Source: CAD feature listing. Evaluate the final solid. Frame: model axes, mm. Face numbers are marked on the shaded views. A direction names the side the tool comes from. Give positions to 0.01 mm unless a question says otherwise; leave off trailing zeros. Loops run counter-clockwise (first coordinate to the right, second up) from the corner with the lowest first, then second, coordinate; pieces in that order, holes last. Notation, with made-up numbers: (46.25, 6) -> (74.25, 6) arc R18 ccw to (74.25, 32) -> close; hole circle Ø5 at (89.5, 66.5). An arc over 180 degrees is marked (long way). Return JSON: item names as keys, results as strings. Group by question number.
(1) Cut plane D-D on z = 14. Give the number of separate pieces and of enclosed holes in the cut face, then the cut area to 3 significant figures.
(2) Cut plane A-A on z = 0. Return loops of the section in (x, y) (3 decimals), then the cut area to 3 significant figures.
(3) Cut plane C-C on z = -3.5. Return loops of the section in (x, y) (3 decimals), then the cut area to 3 significant figures.
(4) Ray query, line 1 (Z direction, x = -13.5, y = 1); line 2 (Z direction, x = -4.5, y = 1); line 3 (Y direction, x = -9, z = 14) (3 decimals). Return the intervals inside material, ascending. Write a range as from..to.
(5) Cut plane B-B on x = 0. Return loops of the section in (y, z) (3 decimals).
(6) Pin query (flat end, axial travel): pin 1 (1.6 mm diameter, centred on x = 3.5, y = 1, fed in from -Z); pin 2 (1.6 mm diameter, centred on x = 13.47, z = 13.47, fed in from -Y); pin 3 (5 mm diameter, centred on x = -2, z = 5, fed in from +Y) (3 decimals). Return the tip coordinate at first contact, or that it passes through.
(7) Access query for the marked faces 1 and 2. Directions: +Z, -Z, +X, -X, +Y, -Y. A direction counts if a zero-diameter tool reaches every point of the face in a straight line with its end or side. Return the directions, or none.
(8) Draft query along X for the marked faces 3, 4 and 5. Return one class per face: released by +X, released by -X, zero draft, split by the parting line, or undercut.
```python
from build123d import *

# Parameters (mm, degrees)
SKETCH1_W                   = 33.528
SKETCH1_H                   = 33.02
BOSS_EXTRUDE1_DEPTH         = 3.175
CUT_EXTRUDE1_DEPTH          = 24.742207585
CUT_EXTRUDE2_DEPTH          = 24.742207585
SKETCH4_W                   = 6.08076
SKETCH4_H                   = 5.45338
BOSS_EXTRUDE2_DEPTH         = 6.08076
SKETCH5_W                   = 6.08076
SKETCH5_H                   = 5.45338
BOSS_EXTRUDE3_DEPTH         = 6.08076
SKETCH6_W                   = 6.08076
SKETCH6_H                   = 5.45338
BOSS_EXTRUDE4_DEPTH         = 6.08076
SKETCH7_W                   = 6.08076
SKETCH7_H                   = 5.45338
BOSS_EXTRUDE5_DEPTH         = 6.08076
HOLE1_D                     = 12.7254
M2_5_CLEARANCE_HOLE1_D      = 2.7051
M3_CLEARANCE_HOLE1_D        = 3.556
M2_5_CLEARANCE_HOLE2_D      = 2.7051
M2_5_CLEARANCE_HOLE2_DEPTH  = 39.60876
M2_5_CLEARANCE_HOLE3_D      = 2.7051
M2_5_CLEARANCE_HOLE3_DEPTH  = 39.60876
M2_5_CLEARANCE_HOLE4_REACH  = 27.061
M2_5_CLEARANCE_HOLE4_BORE_R = 1.35255
FILLET1_R                   = 0.635
FILLET2_R                   = 3.04038
CUT_EXTRUDE3_REACH          = 26.153


with BuildPart() as part:
    # Sketch1 → Boss-Extrude1 (new body)
    with BuildSketch(Plane(origin=(0, 3.175, 0), x_dir=(1, 0, 0), z_dir=(0, 1, 0))):
        Rectangle(SKETCH1_W, SKETCH1_H)
    extrude(amount=-BOSS_EXTRUDE1_DEPTH)

    # Sketch2 → Cut-Extrude1 (cut, through all)
    with BuildSketch(Plane.XZ):
        with BuildLine():
            Line((16.764, -10.42924), (16.764, 10.42924))
            ThreePointArc((16.764, 10.42924), (14.617411383, 9.536940757), (13.7287, 7.388864244))
            Line((13.7287, 7.388864244), (13.7287, -7.388864244))
            ThreePointArc((13.7287, -7.388864244), (14.617411383, -9.536940757), (16.764, -10.42924))
        make_face()
    extrude(amount=-CUT_EXTRUDE1_DEPTH, mode=Mode.SUBTRACT)

    # Sketch3 → Cut-Extrude2 (cut, through all)
    with BuildSketch(Plane.XZ):
        with BuildLine():
            Line((-16.764, 10.42924), (-16.764, -10.42924))
            ThreePointArc((-16.764, -10.42924), (-14.617411383, -9.536940757), (-13.7287, -7.388864244))
            Line((-13.7287, -7.388864244), (-13.7287, 7.388864244))
            ThreePointArc((-13.7287, 7.388864244), (-14.617411383, 9.536940757), (-16.764, 10.42924))
        make_face()
    extrude(amount=-CUT_EXTRUDE2_DEPTH, mode=Mode.SUBTRACT)

    # Sketch4 → Boss-Extrude2 (add)
    with BuildSketch(Plane(origin=(0, 0, -16.51), x_dir=(-1, 0, 0), z_dir=(0, 0, -1))):
        with Locations((13.72362, 5.90169)):
            Rectangle(SKETCH4_W, SKETCH4_H)
    extrude(amount=-BOSS_EXTRUDE2_DEPTH)

    # Sketch5 → Boss-Extrude3 (add)
    with BuildSketch(Plane(origin=(0, 0, -16.51), x_dir=(-1, 0, 0), z_dir=(0, 0, -1))):
        with Locations((-13.72362, 5.90169)):
            Rectangle(SKETCH5_W, SKETCH5_H)
    extrude(amount=-BOSS_EXTRUDE3_DEPTH)

    # Sketch6 → Boss-Extrude4 (add)
    with BuildSketch(Plane.XY.offset(16.51)):
        with Locations((13.72362, 5.90169)):
            Rectangle(SKETCH6_W, SKETCH6_H)
    extrude(amount=-BOSS_EXTRUDE4_DEPTH)

    # Sketch7 → Boss-Extrude5 (add)
    with BuildSketch(Plane.XY.offset(16.51)):
        with Locations((-13.72362, 5.90169)):
            Rectangle(SKETCH7_W, SKETCH7_H)
    extrude(amount=-BOSS_EXTRUDE5_DEPTH)

    # Hole1 (through all)
    with Locations(Plane(origin=(0, 3.175, 0), x_dir=(1, 0, 0), z_dir=(0, 1, 0))):
        with Locations((0, 0)):
            Hole(HOLE1_D / 2)

    # M2.5 Clearance Hole1 (through all)
    with Locations(Plane(origin=(0, 3.175, 0), x_dir=(1, 0, 0), z_dir=(0, 1, 0))):
        with Locations((0, 9.779), (-9.779, 0), (0, -9.779), (9.779, 0)):
            Hole(M2_5_CLEARANCE_HOLE1_D / 2)

    # M3 Clearance Hole1 (through all)
    with Locations(Plane(origin=(0, 3.175, 0), x_dir=(1, 0, 0), z_dir=(0, 1, 0))):
        with Locations((-5.579615818, -13.470384182), (5.579615818, -13.470384182), (5.579615818, 13.470384182), (-5.579615818, 13.470384182), (6.914797213, 6.914797213), (-6.914797213, 6.914797213), (-6.914797213, -6.914797213), (6.914797213, -6.914797213)):
            Hole(M3_CLEARANCE_HOLE1_D / 2)

    # M2.5 Clearance Hole2
    with Locations(Plane(origin=(16.764, 0, 0), x_dir=(0, 0, -1), z_dir=(1, 0, 0))):
        with Locations((-13.470384182, 5.588)):
            Hole(M2_5_CLEARANCE_HOLE2_D / 2, depth=M2_5_CLEARANCE_HOLE2_DEPTH)

    # M2.5 Clearance Hole3
    with Locations(Plane.ZY.offset(16.764)):
        with Locations((-13.470384182, 5.588)):
            Hole(M2_5_CLEARANCE_HOLE3_D / 2, depth=M2_5_CLEARANCE_HOLE3_DEPTH)

    # M2.5 Clearance Hole4 bore → M2.5 Clearance Hole4 (cut, up to next)
    with BuildSketch(Plane(origin=(0, 0, 0), x_dir=(-1, 0, 0), z_dir=(0, -1, 0)), mode=Mode.PRIVATE) as m2_5_clearance_hole4_sk1:
        with Locations((13.470384182, 13.470384182)):
            Circle(M2_5_CLEARANCE_HOLE4_BORE_R)
    m2_5_clearance_hole4_tool1 = extrude(m2_5_clearance_hole4_sk1.sketch, amount=-M2_5_CLEARANCE_HOLE4_REACH, mode=Mode.PRIVATE) & part.part
    # M2.5 Clearance Hole4 bore → M2.5 Clearance Hole4 (cut, up to next)
    with BuildSketch(Plane(origin=(0, 0, 0), x_dir=(-1, 0, 0), z_dir=(0, -1, 0)), mode=Mode.PRIVATE) as m2_5_clearance_hole4_sk2:
        with Locations((-13.470384182, 13.470384182)):
            Circle(M2_5_CLEARANCE_HOLE4_BORE_R)
    m2_5_clearance_hole4_tool2 = extrude(m2_5_clearance_hole4_sk2.sketch, amount=-M2_5_CLEARANCE_HOLE4_REACH, mode=Mode.PRIVATE) & part.part
    # M2.5 Clearance Hole4 bore → M2.5 Clearance Hole4 (cut, up to next)
    with BuildSketch(Plane(origin=(0, 0, 0), x_dir=(-1, 0, 0), z_dir=(0, -1, 0)), mode=Mode.PRIVATE) as m2_5_clearance_hole4_sk3:
        with Locations((-13.470384182, -13.470384182)):
            Circle(M2_5_CLEARANCE_HOLE4_BORE_R)
    m2_5_clearance_hole4_tool3 = extrude(m2_5_clearance_hole4_sk3.sketch, amount=-M2_5_CLEARANCE_HOLE4_REACH, mode=Mode.PRIVATE) & part.part
    # M2.5 Clearance Hole4 bore → M2.5 Clearance Hole4 (cut, up to next)
    with BuildSketch(Plane(origin=(0, 0, 0), x_dir=(-1, 0, 0), z_dir=(0, -1, 0)), mode=Mode.PRIVATE) as m2_5_clearance_hole4_sk4:
        with Locations((13.470384182, -13.470384182)):
            Circle(M2_5_CLEARANCE_HOLE4_BORE_R)
    m2_5_clearance_hole4_tool4 = extrude(m2_5_clearance_hole4_sk4.sketch, amount=-M2_5_CLEARANCE_HOLE4_REACH, mode=Mode.PRIVATE) & part.part
    add(m2_5_clearance_hole4_tool1.solids().sort_by_distance((-13.470384, 0, -13.470384))[0], mode=Mode.SUBTRACT)
    add(m2_5_clearance_hole4_tool2.solids().sort_by_distance((13.470384, 0, -13.470384))[0], mode=Mode.SUBTRACT)
    add(m2_5_clearance_hole4_tool3.solids().sort_by_distance((13.470384, 0, 13.470384))[0], mode=Mode.SUBTRACT)
    add(m2_5_clearance_hole4_tool4.solids().sort_by_distance((-13.470384, 0, 13.470384))[0], mode=Mode.SUBTRACT)

    # Fillet1
    fillet1_edges = [part.edges().sort_by_distance(p)[0] for p in [
        (-16.764, 4.31419, 16.51),
        (-16.764, 4.31419, -16.51),
        (16.764, 4.31419, -16.51),
        (16.764, 4.31419, 16.51),
    ]]
    fillet(fillet1_edges, radius=FILLET1_R)

    # Fillet2
    # the kernel refuses this fillet: 3.04038 mm, written as the material it takes off along each edge
    with BuildSketch(Plane(origin=(-10.68324, 16.22933, -10.42924), x_dir=(-1, 0, 0), z_dir=(0, -1, 0)), Plane(origin=(10.68324, 16.22933, 10.42924), x_dir=(1, 0, 0), z_dir=(0, -1, 0)), Plane(origin=(-10.68324, 3.175, 10.42924), x_dir=(-1, 0, 0), z_dir=(0, 1, 0))) as fillet2_piece_1:
        with BuildLine():
            CenterArc((FILLET2_R, FILLET2_R), FILLET2_R, 180, 90)
            Line((0, FILLET2_R), (0, 0))
            Line((0, 0), (FILLET2_R, 0))
        make_face()
    extrude(amount=13.05433, mode=Mode.SUBTRACT)
    with BuildSketch(Plane(origin=(10.68324, 3.175, -10.42924), x_dir=(0, 0, -1), z_dir=(0, 1, 0))) as fillet2_piece_2:
        with BuildLine():
            CenterArc((FILLET2_R, -FILLET2_R), FILLET2_R, 90, 90)
            Line((0, -FILLET2_R), (0, 0))
            Line((0, 0), (FILLET2_R, 0))
        make_face()
    extrude(amount=13.05433, mode=Mode.SUBTRACT)

    # Sketch20 → Cut-Extrude3 (cut, up to next)
    with BuildSketch(Plane(origin=(0, 3.175, 0), x_dir=(1, 0, 0), z_dir=(0, 1, 0)), mode=Mode.PRIVATE) as cut_extrude3_sk1:
        with BuildLine():
            Line((5.815146261, 9.186050919), (-5.815146261, 9.186050919))
            ThreePointArc((-5.815146261, 9.186050919), (-6.754288773, 9.253077351), (-7.674393598, 9.452797931))
            ThreePointArc((-7.674393598, 9.452797931), (-9.84761666, 10.960236799), (-10.68324, 13.46962))
            Line((-10.68324, 13.46962), (-10.68324, 16.51))
            Line((-10.68324, 16.51), (10.68324, 16.51))
            Line((10.68324, 16.51), (10.68324, 13.46962))
            ThreePointArc((10.68324, 13.46962), (9.84761666, 10.960236799), (7.674393598, 9.452797931))
            ThreePointArc((7.674393598, 9.452797931), (6.754288773, 9.253077351), (5.815146261, 9.186050919))
        make_face()
    cut_extrude3_tool1 = extrude(cut_extrude3_sk1.sketch, amount=-CUT_EXTRUDE3_REACH, mode=Mode.PRIVATE) & part.part
    add(cut_extrude3_tool1.solids().sort_by_distance((0, 3.175, -13.000619))[0], mode=Mode.SUBTRACT)


solid = part.part
```
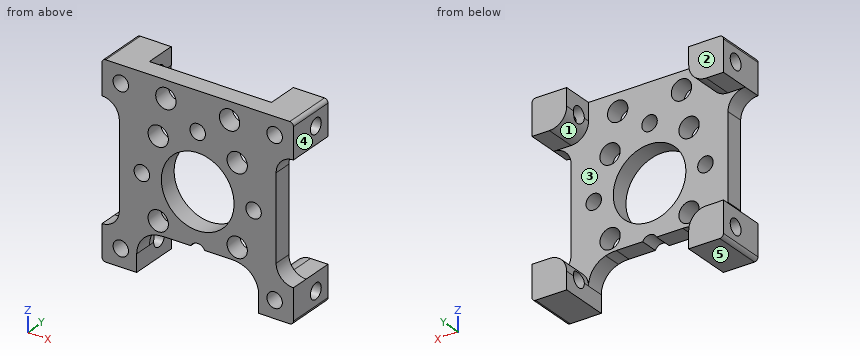
Answers:
{
 "1": {"separate pieces": "7", "enclosed holes": "0", "area": "99.3 mm²"},
 "2": {"outline": "(-13.729, 0) -> (-11.132, 0) -> (-11.132, 3.175) -> (-13.729, 3.175) -> close; (-8.426, 0) -> (-6.363, 0) -> (-6.363, 3.175) -> (-8.426, 3.175) -> close; (6.363, 0) -> (8.426, 0) -> (8.426, 3.175) -> (6.363, 3.175) -> close; (11.132, 0) -> (13.729, 0) -> (13.729, 3.175) -> (11.132, 3.175) -> close", "area": "29.6 mm²"},
 "3": {"outline": "(-13.729, 0) -> (-5.314, 0) -> (-5.314, 3.175) -> (-13.729, 3.175) -> close; (5.314, 0) -> (13.729, 0) -> (13.729, 3.175) -> (5.314, 3.175) -> close", "area": "53.4 mm²"},
 "4": {"line 1": "-16.51..-14.82, -12.12..12.12, 14.82..16.51", "line 2": "-9.19..-4.5, 4.5..12.06, 14.88..16.51", "line 3": "0..3.175"},
 "5": {"outline": "(0, -8.426) -> (3.175, -8.426) -> (3.175, -6.363) -> (0, -6.363) -> close; (0, 6.363) -> (3.175, 6.363) -> (3.175, 8.426) -> (0, 8.426) -> close; (0, 11.132) -> (3.175, 11.132) -> (3.175, 16.51) -> (0, 16.51) -> close"},
 "6": {"pin 1": "z = -9.19", "pin 2": "y = 6.68", "pin 3": "y = 3.175"},
 "7": {"face 1": "+Y", "face 2": "+Z, -Z, +X, -X, +Y"},
 "8": {"face 3": "undercut", "face 4": "released by +X", "face 5": "zero draft"}
}
